Build history of the part. All positions in model axes, mm. A direction names the side the tool comes from. Coordinates: 2 decimals unless noted, no trailing zeros. Loops run counter-clockwise (first coordinate to the right, second up) from the corner with the lowest first, then second, coordinate; pieces in that order, holes last.
Item 1: 3-axis set-ups, long thin cutter, end or side, ignore diameter. For faces 1 (the face through (-51, 0, 4)), 2 (the face through (41, 15, 13)), 3 (the face through (41, 0, 5)), 4 (the face through (41, 0, 20)), 5 (the face through (41, -15, 13)): which of +Z, -Z, +X, -X, +Y, -Y reach the whole face in a straight line?
Item 2: Flat gauge pins, fed straight in: pin 1 (4 mm diameter, centred on x = -48, z = 19, fed in from -Y); pin 2 (6 mm diameter, centred on x = 40, y = 0.5, fed in from -Z); pin 3 (10 mm diameter, centred on x = 39, y = -2.5, fed in from +Z). Where does each tip first touch, or does it go through?
Item 3: Mould opens along X. For faces 6 (the face through (-41, 0, 5)), 7 (the face through (-59, 0, 0)), 8 (the face through (66, 0, 12)) say: released by +X, released by -X, zero draft, split by the parting line, or undercut.
Item 4: Cut at B-B (x = 0). List the corners of the cut face in (y, z), and give its area (3 significant figures).
Item 5: Cut at A-A (y = 0). List the corners of the cut face in (x, z), and give its area (3 significant figures).
Item 6: Drill centre lines: line 1 along X through (y, z) = (27, 8.5); line 2 along Y through (x, z) = (0, 13.75); line 3 along X through (y, z) = (-16.5, 12). Where is each one in solid material? Low to high.
Item 7: Cut at C-C (z = 12.25). List the corners of the cut face in (x, y).
Item 8: Cut at D-D (y = -20.5). List the corners of the cut face in (x, z), and give its area (3 significant figures).
from build123d import *

# Parameters (mm, degrees)
SKETCH1_W           = 60
SKETCH1_H           = 132
BOSS_EXTRUDE1_DEPTH = 25
SKETCH2_W           = 20
SKETCH2_H           = 15
CUT_EXTRUDE1_DEPTH  = 77.68767828
SKETCH4_W           = 20
SKETCH4_H           = 30
CUT_EXTRUDE2_DEPTH  = 5
SKETCH5_W           = 20
SKETCH5_H           = 30
CUT_EXTRUDE3_DEPTH  = 5
SKETCH6_R           = 25
CUT_EXTRUDE4_DEPTH  = 77.68767828


with BuildPart() as part:
    # Sketch1 → Boss-Extrude1 (new body)
    with BuildSketch(Plane(origin=(0, 0, 0), x_dir=(0, 1, 0), z_dir=(0, 0, 1))):
        Rectangle(SKETCH1_W, SKETCH1_H)
    extrude(amount=BOSS_EXTRUDE1_DEPTH)

    # Sketch2 → Cut-Extrude1 (cut, through all)
    with BuildSketch(Plane.XY.offset(25)):
        with Locations((-41, 22.5)):
            Rectangle(SKETCH2_W, SKETCH2_H)
        with Locations((41, 22.5)):
            Rectangle(SKETCH2_W, SKETCH2_H)
        with Locations((41, -22.5)):
            Rectangle(SKETCH2_W, SKETCH2_H)
        with Locations((-41, -22.5)):
            Rectangle(SKETCH2_W, SKETCH2_H)
    extrude(amount=-CUT_EXTRUDE1_DEPTH, mode=Mode.SUBTRACT)

    # Sketch4 → Cut-Extrude2 (cut)
    with BuildSketch(Plane.XY.offset(25)):
        with Locations((-41, 0)):
            Rectangle(SKETCH4_W, SKETCH4_H)
        with Locations((41, 0)):
            Rectangle(SKETCH4_W, SKETCH4_H)
    extrude(amount=-CUT_EXTRUDE2_DEPTH, mode=Mode.SUBTRACT)

    # Sketch5 → Cut-Extrude3 (cut)
    with BuildSketch(Plane(origin=(0, 0, 0), x_dir=(1, 0, 0), z_dir=(0, 0, -1))):
        with Locations((-41, 0)):
            Rectangle(SKETCH5_W, SKETCH5_H)
        with Locations((41, 0)):
            Rectangle(SKETCH5_W, SKETCH5_H)
    extrude(amount=-CUT_EXTRUDE3_DEPTH, mode=Mode.SUBTRACT)

    # Sketch6 → Cut-Extrude4 (cut, through all)
    with BuildSketch(Plane.XY.offset(25)):
        Circle(SKETCH6_R)
    extrude(amount=-CUT_EXTRUDE4_DEPTH, mode=Mode.SUBTRACT)


solid = part.part
Filled sheet:
1. face 1: none
1. face 2: +Z, -Z, +Y
1. face 3: -Z, +Y, -Y
1. face 4: +Z, +Y, -Y
1. face 5: +Z, -Z, -Y
2. pin 1: stops at y = -15
2. pin 2: stops at z = 5
2. pin 3: stops at z = 20
3. face 6: undercut
3. face 7: zero draft
3. face 8: released by +X
4. outline: (-30, 0) - (-25, 0) - (-25, 25) - (-30, 25) - close; (25, 0) - (30, 0) - (30, 25) - (25, 25) - close
4. area: 250 mm2
5. outline: (-66, 0) - (-51, 0) - (-51, 5) - (-31, 5) - (-31, 0) - (-25, 0) - (-25, 25) - (-31, 25) - (-31, 20) - (-51, 20) - (-51, 25) - (-66, 25) - close; (25, 0) - (31, 0) - (31, 5) - (51, 5) - (51, 0) - (66, 0) - (66, 25) - (51, 25) - (51, 20) - (31, 20) - (31, 25) - (25, 25) - close
5. area: 1,650 mm2
6. line 1: x = -66 to -51, -31 to 31, 51 to 66
6. line 2: y = -30 to -25, 25 to 30
6. line 3: x = -66 to -51, -31 to -18.78, 18.78 to 31, 51 to 66
7. outline: (-66, -30) - (-51, -30) - (-51, -15) - (-31, -15) - (-31, -30) - (31, -30) - (31, -15) - (51, -15) - (51, -30) - (66, -30) - (66, 30) - (51, 30) - (51, 15) - (31, 15) - (31, 30) - (-31, 30) - (-31, 15) - (-51, 15) - (-51, 30) - (-66, 30) - close; hole circle Ø50 at (0, 0)
8. outline: (-66, 0) - (-51, 0) - (-51, 25) - (-66, 25) - close; (-31, 0) - (-14.31, 0) - (-14.31, 25) - (-31, 25) - close; (14.31, 0) - (31, 0) - (31, 25) - (14.31, 25) - close; (51, 0) - (66, 0) - (66, 25) - (51, 25) - close
8. area: 1,580 mm2
